from build123d import *

# Parameters (mm, degrees)
FILLET1_R           = 6
SKETCH2_R           = 9
BOSS_EXTRUDE1_DEPTH = 4
SKETCH6_R           = 20
BOSS_EXTRUDE2_DEPTH = 15
SKETCH7_W           = 32.033376833
SKETCH7_H           = 34.641016152
SKETCH7_W_2         = 29.367708721
CUT_EXTRUDE1_DEPTH  = 8.5
CUT_EXTRUDE2_DEPTH  = 8.5
SKETCH10_R          = 7.1
CUT_EXTRUDE3_DEPTH  = 3
FILLET2_R           = 2


with BuildPart() as part:
    # Sketch1 → Revolve1 (revolve)
    with BuildSketch(Plane.XY, mode=Mode.PRIVATE) as revolve1_sk:
        with BuildLine():
            Line((0, 0), (0, 28.5))
            ThreePointArc((0, 28.5), (-9.340770846, 27.226775046), (-18, 23.5))
            Line((-18, 23.5), (-23.9, 6))
            Line((-23.9, 6), (-24.9, 6))
            Line((-24.9, 6), (-24.9, 0))
            Line((-24.9, 0), (0, 0))
        make_face()
    revolve(revolve1_sk.sketch.rotate(Axis((0, 0, 0), (0, 1, 0)), 270), axis=Axis((0, 0, 0), (0, 1, 0)))

    # Fillet1
    fillet1_edges = [part.edges().sort_by_distance(p)[0] for p in [
        (0, 23.5, 18),
    ]]
    fillet(fillet1_edges, radius=FILLET1_R)

    # Sketch2 → Boss-Extrude1 (add)
    with BuildSketch(Plane.XZ):
        with Locations(Location((0, 0, 0), (0, 0, 270))):
            Circle(SKETCH2_R)
    extrude(amount=BOSS_EXTRUDE1_DEPTH)

    # Sketch6 → Boss-Extrude2 (add)
    with BuildSketch(Plane.XZ.offset(4)):
        with Locations(Location((0, 0, 0), (0, 0, 270))):
            Circle(SKETCH6_R)
    extrude(amount=BOSS_EXTRUDE2_DEPTH)

    # Sketch7 → Cut-Extrude1 (cut)
    with BuildSketch(Plane.XZ.offset(19)):
        with Locations((-26.016688417, 0)):
            Rectangle(SKETCH7_W, SKETCH7_H)
        with Locations((24.68385436, 0)):
            Rectangle(SKETCH7_W_2, SKETCH7_H)
    extrude(amount=-CUT_EXTRUDE1_DEPTH, mode=Mode.SUBTRACT)

    # Sketch9 → Cut-Extrude2 (cut)
    with BuildSketch(Plane.XZ.offset(19)):
        with BuildLine():
            Line((-4.728636167, 3), (-27.5, 3))
            Line((-27.5, 3), (-27.5, -3))
            Line((-27.5, -3), (-4.728636167, -3))
            ThreePointArc((-4.728636167, -3), (0, -5.6), (4.728636167, -3))
            Line((4.728636167, -3), (27.5, -3))
            Line((27.5, -3), (27.5, 3))
            Line((27.5, 3), (4.728636167, 3))
            ThreePointArc((4.728636167, 3), (0, 5.6), (-4.728636167, 3))
        make_face()
    extrude(amount=-CUT_EXTRUDE2_DEPTH, mode=Mode.SUBTRACT)

    # Sketch10 → Cut-Extrude3 (cut)
    with BuildSketch(Plane.XZ.offset(19)):
        Circle(SKETCH10_R)
    extrude(amount=-CUT_EXTRUDE3_DEPTH, mode=Mode.SUBTRACT)

    # Fillet2
    fillet2_edges = [part.edges().sort_by_distance(p)[0] for p in [
        (0, -19, 20),
        (5.176380902, -19, -19.318516526),
    ]]
    fillet(fillet2_edges, radius=FILLET2_R)


solid = part.part
Design review of the part built by this model. Coordinates are the model's own, in mm. A direction names the side the tool comes from. Give positions to 0.01 mm unless a question says otherwise; leave off trailing zeros. Write each loop counter-clockwise with the first axis right and the second up, starting at its lowest first coordinate (ties: lowest second). Pieces come first, ordered by that corner, then holes. Notation, with made-up numbers: M -36,19.5 L -24,19.5 A27 cw -24,54.5 Z; hole C 85,42.5 d1. An arc over 180 degrees is marked long. Return JSON: item names as keys, results as strings. Group by question number.
Item 1: The part is to be moulded in two halves that separate along Z. For faces 1 (the conical face through (-5.726, 20.342, -18.184)), 2 (the flat face through (-10, -15, -10)), 3 (the flat face through (7, -15, 3)), say which applies: pulls with the +Z half, pulls with the -Z half, needs draft (parallel to the pull), parting line crosses it, or undercut.
Item 2: Clearance check with flat-ended pins moving along their axes: pin 1 Ø1 at (x, y) = (16.5, 11.5) entering from -Z; pin 2 Ø1.2 at (x, z) = (-2.5, 5.5) entering from -Y; pin 3 Ø4.5 at (y, z) = (-14.5, -8) entering from +X. State where each tip first meets the part, or that it passes through.
Item 3: Take a section at B-B (y = 20). Give the boundary of the cut face in (x, z).
Item 4: Tool access review of faces 4 (the cylindrical face through (2.703, -1.972, -8.584)), 5 (the flat face through (-22.2, 6, -9.3)), 6 (the flat face through (-7, -15, 3)), 7 (the cylindrical face through (0.1, -17.5, 7.1)), 8 (the flat face through (10, -15, 10)): name each direction out of +Z, -Z, +X, -X, +Y, -Y from which nothing blocks a thin tool from reaching the whole face with its end or side.
Item 5: Wall thickness on line 1 along Z through (x, y) = (0, -5); line 2 along X through (y, z) = (-16.5, 5); line 3 along Y through (x, z) = (2, 13.5): over which ranges is each line inside the solid? List them lowest first.
Item 6: Take a section at A-A (y = -14). Give the boundary of the cut face in (x, z).
Return value:
{
 "1": {"face 1": "parting line crosses it", "face 2": "needs draft", "face 3": "undercut"},
 "2": {"pin 1": "stops at z = -15.22", "pin 2": "stops at y = -16", "pin 3": "stops at x = 10"},
 "3": {"outline": "C 0,0 d38.36"},
 "4": {"face 4": "none", "face 5": "+Y", "face 6": "+X, -X, -Y", "face 7": "-Y", "face 8": "+Z, -Z, +X, -Y"},
 "5": {"line 1": "z = -20 to 20", "line 2": "x = -10 to -5.04, 5.04 to 10", "line 3": "y = -19 to -4, 0 to 25.72"},
 "6": {"outline": "M -10,-17.32 A20 ccw 10,-17.32 L 10,-3 L 4.73,-3 A5.6 cw -4.73,-3 L -10,-3 Z; M -10,3 L -4.73,3 A5.6 cw 4.73,3 L 10,3 L 10,17.32 A20 ccw -10,17.32 Z"}
}
